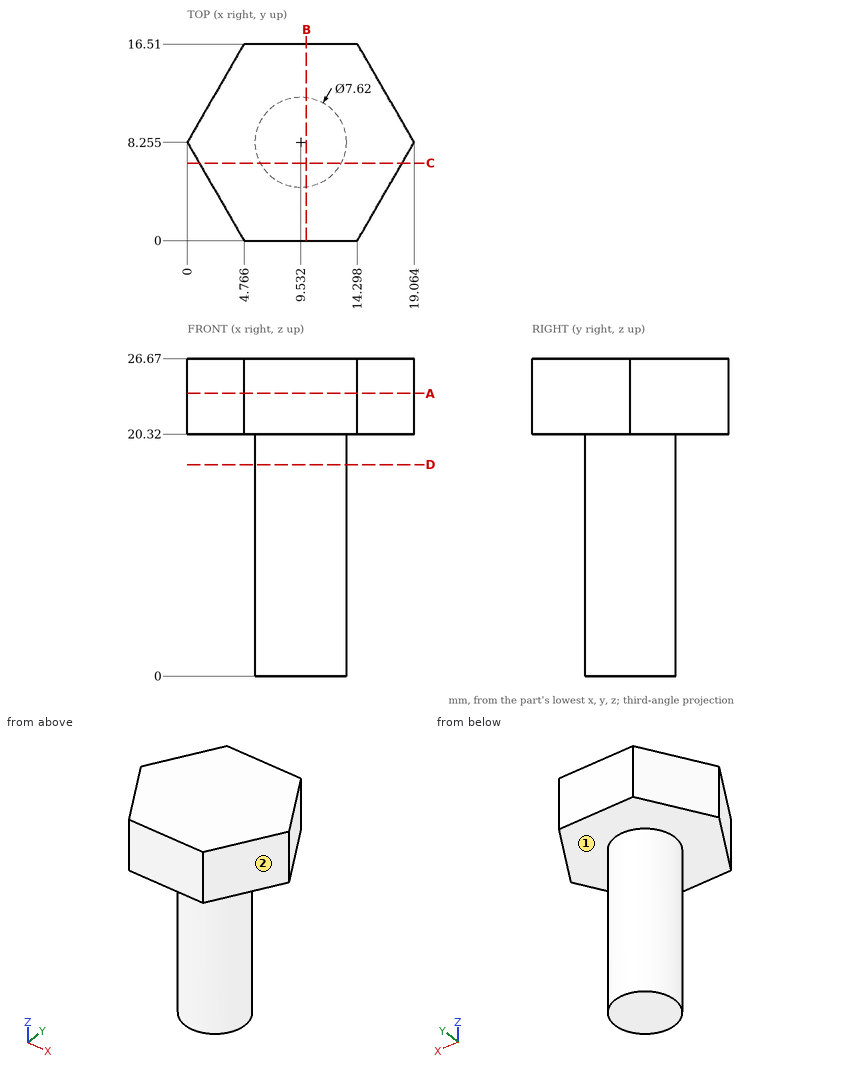
Answer from the drawing. Dimensions are ordinates in mm from the lowest x, y and z of the part. A direction names the side the tool comes from. Round coordinates to 2 decimals unless told otherwise and drop trailing zeros. Loops run counter-clockwise (first coordinate to the right, second up) from the corner with the lowest first, then second, coordinate; pieces in that order, holes last.
1) Consider line 1 (Z direction, x = 7, y = 3.75); line 2 (Y direction, x = 15.5, z = 23.5); line 3 (Y direction, x = 14.5, z = 24). Determine where each line is inside the solid, lowest interval first.
Outcome:
line 1: z = 20.32 to 26.67
line 2: y = 2.08 to 14.43
line 3: y = 0.35 to 16.16
2) A cutting plane is placed at D-D on z = 17.75. Determine the outline of the cut face in (x, y) (3 decimals).
Outcome:
outline: circle Ø7.62 at (9.532, 8.255)
3) For the marked faces 1 and 2, determine the directions among +Z, -Z, +X, -X, +Y, -Y from which every point of the face is accessible in a straight line to the end or side of a thin tool.
Outcome:
face 1: -Z
face 2: +Z, -Z, +X, -Y
4) A cutting plane is placed at B-B on x = 10. Determine the outline of the cut face in (y, z).
Outcome:
outline: (0, 20.32) - (4.47, 20.32) - (4.47, 0) - (12.04, 0) - (12.04, 20.32) - (16.51, 20.32) - (16.51, 26.67) - (0, 26.67) - close
5) A cutting plane is placed at C-C on y = 6.5. Determine the outline of the cut face in (x, z).
Outcome:
outline: (1.01, 20.32) - (6.15, 20.32) - (6.15, 0) - (12.91, 0) - (12.91, 20.32) - (18.05, 20.32) - (18.05, 26.67) - (1.01, 26.67) - close
6) Given P1, Ø6, axis at y = 7, z = 5, coming from the +X side; P2, Ø5, axis at y = 5, z = 19, coming from the -X side; P3, Ø5, axis at y = 3.5, z = 22, coming from the +X side, each flat-ended and moving along its own axis, determine where each tip first touches the part or whether it passes through.
Outcome:
P1: stops at x = 13.34
P2: stops at x = 0.65
P3: stops at x = 17.76
7) A cutting plane is placed at A-A on z = 23.75. Determine the outline of the cut face in (x, y) (3 decimals).
Outcome:
outline: (0, 8.255) - (4.766, 0) - (14.298, 0) - (19.064, 8.255) - (14.298, 16.51) - (4.766, 16.51) - close
